from build123d import *

# Parameters (mm, degrees)
SKETCH1_W                                        = 46
SKETCH1_H                                        = 36
BOSS_EXTRUDE1_DEPTH                              = 4
CBORE_FOR_M2_PAN_HEAD_MACHINE_SCREW1_D           = 2.4
CBORE_FOR_M2_PAN_HEAD_MACHINE_SCREW1_CBORE_D     = 5
CBORE_FOR_M2_PAN_HEAD_MACHINE_SCREW1_CBORE_DEPTH = 2.6
SKETCH6_W                                        = 47
SKETCH6_H                                        = 36
BOSS_EXTRUDE2_DEPTH                              = 4
SKETCH7_R                                        = 4
BOSS_EXTRUDE3_DEPTH                              = 7
CUT_EXTRUDE3_DEPTH                               = 6.5
FILLET3_R                                        = 4
SKETCH13_W                                       = 14
SKETCH13_H                                       = 28
CUT_EXTRUDE5_DEPTH                               = 27
SKETCH16_W                                       = 14
SKETCH16_H                                       = 7
BOSS_EXTRUDE4_DEPTH                              = 4
SKETCH17_W                                       = 10
SKETCH17_H                                       = 10
CUT_EXTRUDE6_DEPTH                               = 10
FILLET4_R                                        = 1.5
CBORE_START                                      = 36.211611197
CBORE_FOR_M2_PAN_HEAD_MACHINE_SCREW2_OUT_R       = 2.5
CBORE_FOR_M2_PAN_HEAD_MACHINE_SCREW2_DEPTH       = 2.6
CBORE_START_2                                    = 34.811611197
CBORE_FOR_M2_PAN_HEAD_MACHINE_SCREW2_2_O_R       = 1.2
CBORE_FOR_M2_PAN_HEAD_MACHINE_SCREW2_2_DEPTH     = 1.4


# Read off the part's stored shape, not the designer's step: CBORE for M2 Pan Head Machine Screw2
with BuildPart() as part:
    # Sketch1 → Boss-Extrude1 (new body)
    with BuildSketch(Plane(origin=(0, 0, 34.811611197), x_dir=(-1, 0, 0), z_dir=(0, 0, -1))):
        Rectangle(SKETCH1_W, SKETCH1_H)
    extrude(amount=-BOSS_EXTRUDE1_DEPTH)

    # CBORE for M2 Pan Head Machine Screw1 (through all)
    with Locations(Plane(origin=(0, 0, 34.811611197), x_dir=(-1, 0, 0), z_dir=(0, 0, -1))):
        with Locations((12, -8), (-18, -8), (-18, 8), (12, 8)):
            CounterBoreHole(CBORE_FOR_M2_PAN_HEAD_MACHINE_SCREW1_D / 2, CBORE_FOR_M2_PAN_HEAD_MACHINE_SCREW1_CBORE_D / 2, CBORE_FOR_M2_PAN_HEAD_MACHINE_SCREW1_CBORE_DEPTH)

    # Sketch6 → Boss-Extrude2 (add)
    with BuildSketch(Plane.XY.offset(38.811611197)):
        with Locations((-46.5, 0)):
            Rectangle(SKETCH6_W, SKETCH6_H)
    extrude(amount=-BOSS_EXTRUDE2_DEPTH)

    # Sketch7 → Boss-Extrude3 (add)
    with BuildSketch(Plane.XY.offset(38.811611197)):
        with Locations(Location((-66, 14, 0), (0, 0, 180))):
            Circle(SKETCH7_R)
        with Locations(Location((-29, 14, 0), (0, 0, 90))):
            Circle(SKETCH7_R)
        with Locations(Location((-66, -14, 0), (0, 0, 180))):
            Circle(SKETCH7_R)
        with Locations(Location((-29, -14, 0), (0, 0, 270))):
            Circle(SKETCH7_R)
    extrude(amount=BOSS_EXTRUDE3_DEPTH)

    # Sketch10 → Cut-Extrude3 (cut)
    with BuildSketch(Plane.XY.offset(45.811611197)):
        Polygon((-64.556624327, 16.5), (-67.443375673, 16.5), (-68.886751346, 14), (-67.443375673, 11.5), (-64.556624327, 11.5), (-63.113248654, 14), align=None)
        Polygon((-64.556624327, -11.5), (-67.443375673, -11.5), (-68.886751346, -14), (-67.443375673, -16.5), (-64.556624327, -16.5), (-63.113248654, -14), align=None)
        Polygon((-27.556624327, 16.5), (-30.443375673, 16.5), (-31.886751346, 14), (-30.443375673, 11.5), (-27.556624327, 11.5), (-26.113248654, 14), align=None)
        Polygon((-27.556624327, -11.5), (-30.443375673, -11.5), (-31.886751346, -14), (-30.443375673, -16.5), (-27.556624327, -16.5), (-26.113248654, -14), align=None)
    extrude(amount=-CUT_EXTRUDE3_DEPTH, mode=Mode.SUBTRACT)

    # Fillet3
    fillet3_edges = [part.edges().sort_by_distance(p)[0] for p in [
        (-70, -18, 36.811611197),
        (23, -18, 36.811611197),
        (23, 18, 36.811611197),
        (-70, 18, 36.811611197),
    ]]
    fillet(fillet3_edges, radius=FILLET3_R)

    # Sketch13 → Cut-Extrude5 (cut)
    with BuildSketch(Plane.XY.offset(38.811611197)):
        with Locations((1.5, 0)):
            Rectangle(SKETCH13_W, SKETCH13_H)
    extrude(amount=-CUT_EXTRUDE5_DEPTH, mode=Mode.SUBTRACT)

    # Sketch16 → Boss-Extrude4 (add)
    with BuildSketch(Plane.XY.offset(38.811611197)):
        with Locations((1.5, 0)):
            Rectangle(SKETCH16_W, SKETCH16_H)
    extrude(amount=-BOSS_EXTRUDE4_DEPTH)

    # Sketch17 → Cut-Extrude6 (cut)
    with BuildSketch(Plane.XY.offset(38.811611197)):
        with Locations((-20, 0)):
            Rectangle(SKETCH17_W, SKETCH17_H)
    extrude(amount=-CUT_EXTRUDE6_DEPTH, mode=Mode.SUBTRACT)

    # Fillet4
    fillet4_edges = [part.edges().sort_by_distance(p)[0] for p in [
        (-5.5, 14, 36.811611197),
        (8.5, 14, 36.811611197),
        (8.5, -14, 36.811611197),
        (-5.5, -14, 36.811611197),
        (8.5, -3.5, 36.811611197),
        (8.5, 3.5, 36.811611197),
        (-5.5, 3.5, 36.811611197),
        (-5.5, -3.5, 36.811611197),
        (-25, -5, 36.811611197),
        (-25, 5, 36.811611197),
        (-15, 5, 36.811611197),
        (-15, -5, 36.811611197),
    ]]
    fillet(fillet4_edges, radius=FILLET4_R)

    # CBORE for M2 Pan Head Machine Screw2 out → CBORE for M2 Pan Head Machine Screw2 (cut)
    with BuildSketch(Plane.XY.offset(CBORE_START)):
        with Locations((-58.75, 14)):
            Circle(CBORE_FOR_M2_PAN_HEAD_MACHINE_SCREW2_OUT_R)
        with Locations((11.75, -14)):
            Circle(CBORE_FOR_M2_PAN_HEAD_MACHINE_SCREW2_OUT_R)
        with Locations((-58.75, -14)):
            Circle(CBORE_FOR_M2_PAN_HEAD_MACHINE_SCREW2_OUT_R)
        with Locations((11.75, 14)):
            Circle(CBORE_FOR_M2_PAN_HEAD_MACHINE_SCREW2_OUT_R)
    extrude(amount=CBORE_FOR_M2_PAN_HEAD_MACHINE_SCREW2_DEPTH, mode=Mode.SUBTRACT)

    # CBORE for M2 Pan Head Machine Screw2 2 o → CBORE for M2 Pan Head Machine Screw2 2 (cut)
    with BuildSketch(Plane.XY.offset(CBORE_START_2)):
        with Locations((-58.75, 14)):
            Circle(CBORE_FOR_M2_PAN_HEAD_MACHINE_SCREW2_2_O_R)
        with Locations((11.75, -14)):
            Circle(CBORE_FOR_M2_PAN_HEAD_MACHINE_SCREW2_2_O_R)
        with Locations((-58.75, -14)):
            Circle(CBORE_FOR_M2_PAN_HEAD_MACHINE_SCREW2_2_O_R)
        with Locations((11.75, 14)):
            Circle(CBORE_FOR_M2_PAN_HEAD_MACHINE_SCREW2_2_O_R)
    extrude(amount=CBORE_FOR_M2_PAN_HEAD_MACHINE_SCREW2_2_DEPTH, mode=Mode.SUBTRACT)


solid = part.part
Design review of the part built by this model. Coordinates are the model's own, in mm. A direction names the side the tool comes from. Round coordinates to 2 decimals unless told otherwise and drop trailing zeros. Write each loop counter-clockwise with the first axis right and the second up, starting at its lowest first coordinate (ties: lowest second). Pieces come first, ordered by that corner, then holes. Notation, with made-up numbers: (-3.5, 50.5) -> (52.5, 50.5) arc R19 ccw to (52.5, 55.5) -> close; hole circle Ø3 at (-21.75, -2). An arc over 180 degrees is marked (long way). One line per item, written item: value. Start each with the question number.
Q1. Add section C-C (x = 18). Give the boundary of the cut face in (y, z).
Q2. Add section A-A (z = 44). Give the boundary of the cut face in (x, y).
Q3. To check wall thickness, follow probe 1 along Y at (x, z) = (11.75, 37.7); probe 2 along Y at (x, z) = (18, 36); probe 3 along Z at (x, y) = (-19, 6.5). State the ranges of each line that lie inside material, in increasing order.
Q4. Insertion check: P1, Ø3, axis at x = 18, y = 8, coming from the +Z side; P2, Ø2.5, axis at x = -12.5, y = 7, coming from the -Z side; P3, Ø4.5, axis at x = -58.75, y = 14, coming from the +Z side; P4, Ø1.4, axis at x = -58.75, y = -14, coming from the -Z side. Each pin has a flat end and moves straight along its axis. Give the tip position at first contact, or say it passes through.
Q5. Add section B-B (y = -8). Give the boundary of the cut face in (x, z), then the cut area to 3 significant figures.
Q6. Tool access review of faces 1 (the face through (1, 14, 37)), 2 (the face through (-56.44, -14.96, 37.49)), 3 (the face through (-66, 17, 45.812)): name each direction out of +Z, -Z, +X, -X, +Y, -Y from which nothing blocks a thin tool from reaching the whole face with its end or side.
Q7. The part is to be moulded in two halves that separate along Y. For faces 4 (the face through (9.766, -15.521, 37.493)), 5 (the face through (-66, -11, 45.812)), say which applies: pulls with the +Y half, pulls with the -Y half, needs draft (parallel to the pull), parting line crosses it, or undercut.
Q8. Add section D-D (x = 5.5). Give the boundary of the cut face in (y, z).
Response:
1. outline: (-18, 34.81) -> (-10.5, 34.81) -> (-10.5, 37.41) -> (-9.2, 37.41) -> (-9.2, 38.81) -> (-18, 38.81) -> close; (-6.8, 37.41) -> (-5.5, 37.41) -> (-5.5, 34.81) -> (5.5, 34.81) -> (5.5, 37.41) -> (6.8, 37.41) -> (6.8, 38.81) -> (-6.8, 38.81) -> close; (9.2, 37.41) -> (10.5, 37.41) -> (10.5, 34.81) -> (18, 34.81) -> (18, 38.81) -> (9.2, 38.81) -> close
2. outline: circle Ø8 at (-66, -14); circle Ø8 at (-66, 14); circle Ø8 at (-29, -14); circle Ø8 at (-29, 14); hole (-68.89, -14) -> (-67.44, -16.5) -> (-64.56, -16.5) -> (-63.11, -14) -> (-64.56, -11.5) -> (-67.44, -11.5) -> close; hole (-68.89, 14) -> (-67.44, 11.5) -> (-64.56, 11.5) -> (-63.11, 14) -> (-64.56, 16.5) -> (-67.44, 16.5) -> close; hole (-31.89, -14) -> (-30.44, -16.5) -> (-27.56, -16.5) -> (-26.11, -14) -> (-27.56, -11.5) -> (-30.44, -11.5) -> close; hole (-31.89, 14) -> (-30.44, 11.5) -> (-27.56, 11.5) -> (-26.11, 14) -> (-27.56, 16.5) -> (-30.44, 16.5) -> close
3. probe 1: y = -18 to -16.5, -11.5 to 11.5, 16.5 to 18
3. probe 2: y = -18 to -10.5, -5.5 to 5.5, 10.5 to 18
3. probe 3: z = 34.81 to 38.81
4. P1: stops at z = 38.81
4. P2: stops at z = 37.41
4. P3: stops at z = 36.21
4. P4: passes through
5. outline: (-70, 34.81) -> (-14.5, 34.81) -> (-14.5, 37.41) -> (-13.2, 37.41) -> (-13.2, 38.81) -> (-70, 38.81) -> close; (-10.8, 37.41) -> (-9.5, 37.41) -> (-9.5, 34.81) -> (-5.5, 34.81) -> (-5.5, 38.81) -> (-10.8, 38.81) -> close; (8.5, 34.81) -> (15.5, 34.81) -> (15.5, 37.41) -> (16.8, 37.41) -> (16.8, 38.81) -> (8.5, 38.81) -> close; (19.2, 37.41) -> (20.5, 37.41) -> (20.5, 34.81) -> (23, 34.81) -> (23, 38.81) -> (19.2, 38.81) -> close
5. area: 283 mm^2
6. face 1: +Z, -Z
6. face 2: +Z
6. face 3: +Z, +X, -X, +Y, -Y
7. face 4: undercut
7. face 5: needs draft
8. outline: (-18, 34.81) -> (-14, 34.81) -> (-14, 38.81) -> (-18, 38.81) -> close; (-3.5, 34.81) -> (3.5, 34.81) -> (3.5, 38.81) -> (-3.5, 38.81) -> close; (14, 34.81) -> (18, 34.81) -> (18, 38.81) -> (14, 38.81) -> close
